Autodesk Inventor part; units mm, degrees
ref_plane "YZ Plane" through (0, 0, 0) normal (1, 0, 0) x (0, 1, 0)
ref_plane "XZ Plane" through (0, 0, 0) normal (0, 1, 0) x (-1, 0, 0)
ref_plane "XY Plane" through (0, 0, 0) normal (0, 0, 1) x (1, 0, 0)
sketch "Esquisse1" plane through (0, 0, 0) normal (1, 0, 0) x (0, 1, 0)
  line L0 (0, 0) -> (0, -6.3939)
  line L1 (9.5, 0) -> (2.05, 0)
  line L2 (9.5, 0) -> (9.5, -1.5)
  line L3 (9.5, -1.5) -> (8, -1.5)
  line L4 (8, -1.5) -> (8, -3.5)
  line L5 (8, -3.5) -> (7, -3.5)
  line L6 (2.05, 0) -> (2.05, -3)
  line L7 (7, -3.5) -> (5.5, -3)
  line L8 (5.5, -3) -> (2.05, -3)
  dimension "d1" = 1.5
  dimension "d2" = 1.5
  dimension "d4" = 16
  dimension "d5" = 4.1
  dimension "d10" = 2
  dimension "d11" = 3
  dimension "d12" = 1.5
  dimension "d13" = 1
revolve "Révolution1" add sketch "Esquisse1" angle 360 about axis through (0, 0, 0) along (0, 0, -1)
sketch "Esquisse2" plane through (0, 0, 0) normal (0, 0, 1) x (1, 0, 0)
  line L0 (4.6188, 8) -> (9.2376, 0)
  line L1 (9.2376, 0) -> (4.6188, -8)
  line L2 (4.6188, -8) -> (-4.6188, -8)
  line L3 (-4.6188, -8) -> (-9.2376, 0)
  line L4 (-9.2376, 0) -> (-4.6188, 8)
  line L5 (-4.6188, 8) -> (4.6188, 8)
  circle A0 centre (0, 0) radius 9.5
  dimension "d7" = 16
extrude "Extrusion1" cut sketch "Esquisse2" against normal up to surface (1.5 mm away)
thread "Filetage1"
properties part number "cartridge_locker_piston_top"
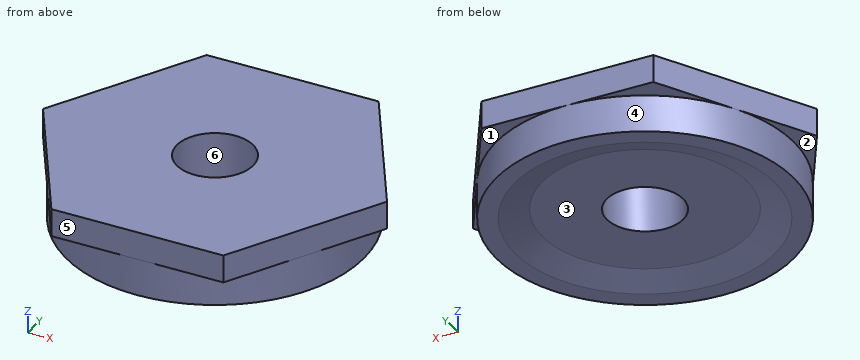
Could you check a few things on this model? Use its own coordinates, in mm. Face numbers are marked on the shaded views. A direction names the side the tool comes from. Give positions to 0.01 mm unless a question says otherwise; leave off trailing zeros. Write each loop counter-clockwise with the first axis right and the second up, starting at its lowest first coordinate (ties: lowest second). Pieces come first, ordered by that corner, then holes. Notation, with made-up numbers: (78.25, 69) -> (110.25, 69) arc R16 ccw to (110.25, 80) -> close; hole circle Ø1 at (-7, 1.25). An arc over 180 degrees is marked (long way). Answer as a JSON object with one key per item and string values.
Q1. Which directions (+Z, -Z, +X, -X, +Y, -Y) give clear straight access to the entire face, cutting with the end or side of a thin tool? Please do the marked faces 1, 2 and 3.
Taken from the geometry:
{"face 1": "-Z, +X, +Y", "face 2": "-Z, -X", "face 3": "-Z"}
Q2. Will these pins go through, and if not, where does the flat tip stop? pin 1 Ø5.5 at (x, y) = (0, 0) entering from -Z; pin 2 Ø2 at (x, y) = (-2, 5.5) entering from -Z; pin 3 Ø1.5 at (y, z) = (5, -1) entering from -X.
Taken from the geometry:
{"pin 1": "stops at z = -3", "pin 2": "stops at z = -3.45", "pin 3": "stops at x = -6.78"}
Q3. Suppose I cut it at A-A on z = -0.25. Write out the boundary of the cut face in (x, y), then the cut area to 4 significant figures.
Taken from the geometry:
{"outline": "(-9.24, 0) -> (-4.62, -8) -> (4.62, -8) -> (9.24, 0) -> (4.62, 8) -> (-4.62, 8) -> close; hole circle Ø4.1 at (0, 0)", "area": "208.5 mm²"}
Q4. Suppose I cut it at B-B on z = -3.2. Write out the boundary of the cut face in (x, y), then the cut area to 3 significant figures.
Taken from the geometry:
{"outline": "circle Ø16 at (0, 0); hole circle Ø12.2 at (0, 0)", "area": "84.2 mm²"}
Q5. Please list where these lines run through material, in increasing order: L1, parallel to Z at x = 0.75, y = -2.5; L2, parallel to X at y = 0, z = -1.6; L3, parallel to X at y = -1, z = -0.65.
Taken from the geometry:
{"L1": "z = -3 to 0", "L2": "x = -8 to -2.05, 2.05 to 8", "L3": "x = -8.66 to -1.79, 1.79 to 8.66"}
Q6. We'd pull the mould along X, two halves only. Please class the marked faces 4, 5 and 6: released by +X, released by -X, zero draft, split by the parting line, or undercut.
Taken from the geometry:
{"face 4": "split by the parting line", "face 5": "zero draft", "face 6": "undercut"}
